from build123d import *

# Parameters (mm, degrees)
BOSS_EXTRUDE1_DEPTH   = 20
F_6_CLEARANCE_HOLE1_D = 3.7973
F_1_CLEARANCE_HOLE2_D = 2.0574
F_6_CLEARANCE_HOLE2_D = 3.7973


with BuildPart() as part:
    # Sketch2 → Boss-Extrude1 (new body)
    with BuildSketch(Plane.XY):
        Polygon((0, 0), (0, 87.1), (40, 87.1), (40, 85.5125), (1.5875, 85.5125), (1.5875, 0), align=None)
    extrude(amount=BOSS_EXTRUDE1_DEPTH)

    # #6 Clearance Hole1 (through all)
    with Locations(Plane(origin=(0, 87.1, 0), x_dir=(1, 0, 0), z_dir=(0, 1, 0))):
        with Locations((10, -10), (30, -10)):
            Hole(F_6_CLEARANCE_HOLE1_D / 2)

    # #1 Clearance Hole2 (through all)
    with Locations(Plane.ZY):
        with Locations((10, 10), (10, 28.2)):
            Hole(F_1_CLEARANCE_HOLE2_D / 2)

    # #6 Clearance Hole2 (through all)
    with Locations(Plane.ZY):
        with Locations((10, 43.2)):
            Hole(F_6_CLEARANCE_HOLE2_D / 2)


solid = part.part
Part model, mm, in its own coordinate system. A direction names the side the tool comes from. Coordinates: 2 decimals unless noted, no trailing zeros. Loops run counter-clockwise (first coordinate to the right, second up) from the corner with the lowest first, then second, coordinate; pieces in that order, holes last. Notation, with made-up numbers: (19, 59.25) -> (75, 59.25) arc R14 cw to (75, 71.25) -> close; hole circle Ø4 at (50, 59). An arc over 180 degrees is marked (long way). Use a Markdown table: item, result. Add a question column.
Item 1: Band-saw the part on A-A on z = 10. Write the cut outline in (x, y).
Item 2: Band-saw the part on D-D on z = 6.5. Write the cut outline in (x, y).
Item 3: Band-saw the part on C-C on x = 30. Write the cut outline in (y, z).
Item 4: Which spindle directions (+Z, -Z, +X, -X, +Y, -Y) get a long thin tool onto all of the face, cutting with end or side? Do faces 1 (the flat face through (0, 42.9, 12.1)), 2 (the flat face through (21, 85.512, 10)). Say none if no direction does.
Item 5: Flat gauge pins, fed straight in: P1, Ø3.5, axis at y = 28.2, z = 10, coming from the +X side; P2, Ø6, axis at x = 13, z = 7.5, coming from the -Y side. Where does each tip first touch, or does it go through?
Item 6: Pull direction Z, two halves, no side cores. Call faces 3 (the flat face through (1, 63, 0)), 4 (the cylindrical face through (0.8, 27.3, 9.5)), 5 (the flat face through (1, 63, 20)): +Z half, -Z half, draft (parallel to the pull), parting line (faces both ways), or undercut.
Item 7: Band-saw the part on B-B on y = 43.2. Write the cut outline in (x, z).
Item 8: Probe probe 1 along Y at (x, z) = (0.9, 10); probe 2 along X at (y, z) = (85.9, 10); probe 3 along Z at (x, y) = (1, 28). List the from-to ranges inside material, lowest first.
Geometry says:
| question | item | result |
|---|---|---|
| 1 | outline | (0, 0) -> (1.59, 0) -> (1.59, 8.97) -> (0, 8.97) -> close; (0, 11.03) -> (1.59, 11.03) -> (1.59, 27.17) -> (0, 27.17) -> close; (0, 29.23) -> (1.59, 29.23) -> (1.59, 41.3) -> (0, 41.3) -> close; (0, 45.1) -> (1.59, 45.1) -> (1.59, 85.51) -> (8.1, 85.51) -> (8.1, 87.1) -> (0, 87.1) -> close; (11.9, 85.51) -> (28.1, 85.51) -> (28.1, 87.1) -> (11.9, 87.1) -> close; (31.9, 85.51) -> (40, 85.51) -> (40, 87.1) -> (31.9, 87.1) -> close |
| 2 | outline | (0, 0) -> (1.59, 0) -> (1.59, 85.51) -> (40, 85.51) -> (40, 87.1) -> (0, 87.1) -> close |
| 3 | outline | (85.51, 0) -> (87.1, 0) -> (87.1, 8.1) -> (85.51, 8.1) -> close; (85.51, 11.9) -> (87.1, 11.9) -> (87.1, 20) -> (85.51, 20) -> close |
| 4 | face 1 | +Z, -Z, -X, +Y, -Y |
| 4 | face 2 | +Z, -Z, +X, -Y |
| 5 | P1 | x = 1.59 |
| 5 | P2 | y = 85.51 |
| 6 | face 3 | -Z half |
| 6 | face 4 | undercut |
| 6 | face 5 | +Z half |
| 7 | outline | (0, 0) -> (1.59, 0) -> (1.59, 8.1) -> (0, 8.1) -> close; (0, 11.9) -> (1.59, 11.9) -> (1.59, 20) -> (0, 20) -> close |
| 8 | probe 1 | 0 to 8.97, 11.03 to 27.17, 29.23 to 41.3, 45.1 to 87.1 |
| 8 | probe 2 | 0 to 8.1, 11.9 to 28.1, 31.9 to 40 |
| 8 | probe 3 | 0 to 8.99, 11.01 to 20 |
